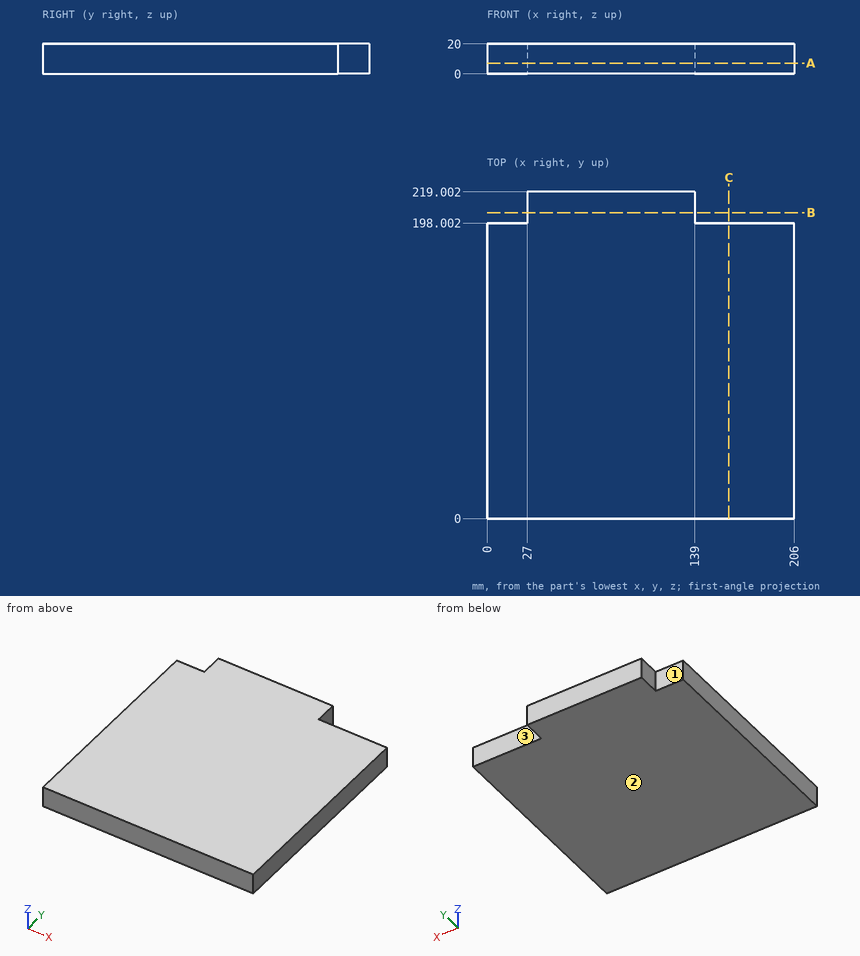
Here's the drawing with two shaded views (mm, measured from the low corner). I have some questions. A direction names the side the tool comes from. Give positions to 0.01 mm unless a question says otherwise; leave off trailing zeros. Write each loop counter-clockwise with the first axis right and the second up, starting at its lowest first coordinate (ties: lowest second). Pieces come first, ordered by that corner, then holes. Notation, with made-up numbers: (-2.75, 81.5) -> (30.25, 81.5) arc R18 cw to (30.25, 115.5) -> close; hole circle Ø8 at (25.25, 1). An arc over 180 degrees is marked (long way). Answer as a JSON object with one key per item and string values. Group by question number.
Item 1: Suppose I cut it at A-A (z = 7.25). Please give me the cut outline in (x, y), plus the area to 3 significant figures.
Item 2: I'm going to push flat-ended pins straight in: P1, Ø6, axis at y = 208.5, z = 10.5, coming from the -X side; P2, Ø6, axis at y = 209, z = 11, coming from the +X side; P3, Ø8, axis at x = 167.5, z = 7, coming from the +Y side. Where does each tip first touch, or does it pass through?
Item 3: Suppose I cut it at B-B (y = 205). Please give me the cut outline in (x, z).
Item 4: For the marked faces 1, 2 and 3, which set-ups out of +Z, -Z, +X, -X, +Y, -Y let a thin tool reach every point of the face, with its end or its side?
Item 5: Suppose I cut it at C-C (x = 162). Please give me the cut outline in (y, z), plus the area to 3 significant figures.
Item 6: Please list where these lines run through material, in increasing order: line 1 (X direction, y = 201, z = 17.5); line 2 (Y direction, x = 189, z = 4.25). Write a range as [from, to].
Findings:
{
 "1": {"outline": "(0, 0) -> (206, 0) -> (206, 198) -> (139, 198) -> (139, 219) -> (27, 219) -> (27, 198) -> (0, 198) -> close", "area": "43,100 mm²"},
 "2": {"P1": "stops at x = 27", "P2": "stops at x = 139", "P3": "stops at y = 198"},
 "3": {"outline": "(27, 0) -> (139, 0) -> (139, 20) -> (27, 20) -> close"},
 "4": {"face 1": "+Z, -Z, -X, +Y", "face 2": "-Z, +X, -X, +Y, -Y", "face 3": "+Z, -Z, +X, +Y"},
 "5": {"outline": "(0, 0) -> (198, 0) -> (198, 20) -> (0, 20) -> close", "area": "3,960 mm²"},
 "6": {"line 1": "x = [27, 139]", "line 2": "y = [0, 198]"}
}
